Part print with two shaded views. Sizes in mm from the minimum x, y, z corner. Round coordinates to 2 decimals unless told otherwise and drop trailing zeros. Loops run counter-clockwise (first coordinate to the right, second up) from the corner with the lowest first, then second, coordinate; pieces in that order, holes last. Notation, with made-up numbers: (-2.5, 50.25) -> (39.5, 50.25) arc R24 cw to (39.5, 72.25) -> close; hole circle Ø8 at (-38.5, 41). An arc over 180 degrees is marked (long way). Use a Markdown table: item, result. Add a question column.
Item 1: Cut at C-C, the plane z = 1. List the corners of the cut face in (x, y).
Item 2: Flat gauge pin, fed straight in: pin 1 (3 mm diameter, centred on y = 2, z = 2, fed in from +X). Where does the tip first touch, or does it go through?
Item 3: Probe line 1 (Z direction, x = 4, y = 1.3); line 2 (X direction, y = 4.35, z = 4.75); line 3 (X direction, y = 3.95, z = 4.5). List the from-to ranges inside material, lowest first. Write a range as [from, to].
Item 4: Cut at B-B, the plane y = 3.8. List the corners of the cut face in (x, z).
Item 5: Cut at A-A, the plane z = 5. List the corners of the cut face in (x, y).
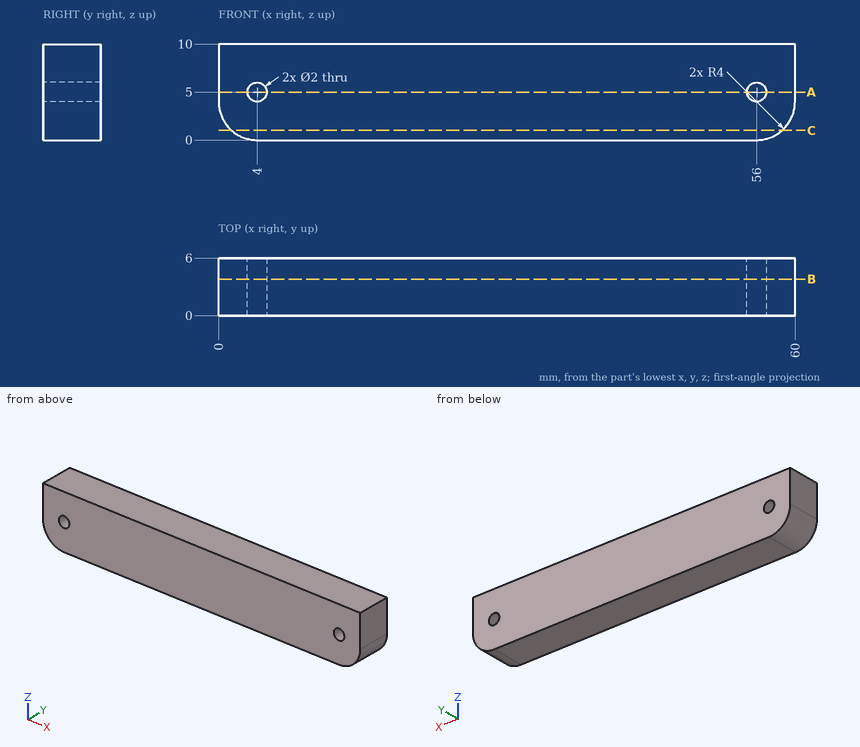
A:
| question | item | result |
|---|---|---|
| 1 | outline | (1.35, 0) -> (58.65, 0) -> (58.65, 6) -> (1.35, 6) -> close |
| 2 | pin 1 | stops at x = 59.97 |
| 3 | line 1 | z = [0, 4], [6, 10] |
| 3 | line 2 | x = [0, 3.03], [4.97, 55.03], [56.97, 60] |
| 3 | line 3 | x = [0, 3.13], [4.87, 55.13], [56.87, 60] |
| 4 | outline | (0, 4) arc R4 ccw to (4, 0) -> (56, 0) arc R4 ccw to (60, 4) -> (60, 10) -> (0, 10) -> close; hole circle Ø2 at (4, 5); hole circle Ø2 at (56, 5) |
| 5 | outline | (0, 0) -> (3, 0) -> (3, 6) -> (0, 6) -> close; (5, 0) -> (55, 0) -> (55, 6) -> (5, 6) -> close; (57, 0) -> (60, 0) -> (60, 6) -> (57, 6) -> close |
